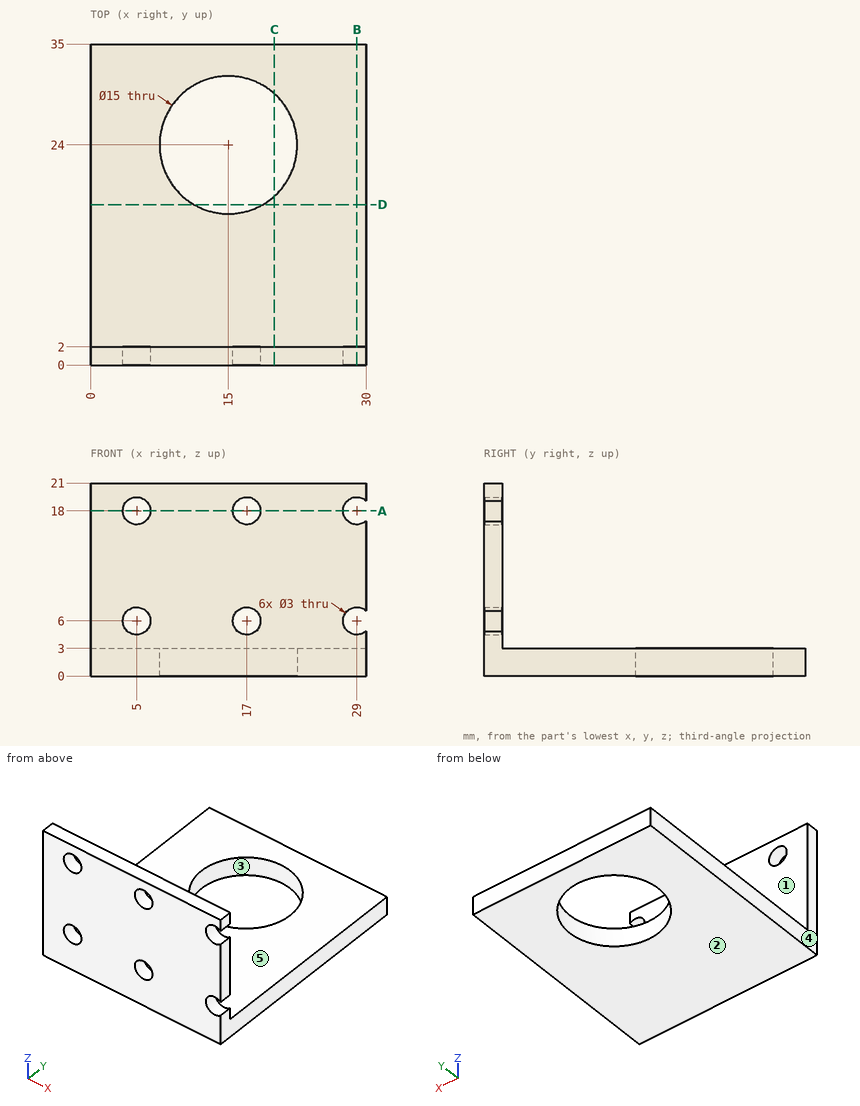
Print and shaded views of the part. All mm, measured from the part's lowest x, y and z. A direction names the side the tool comes from. Round coordinates to 2 decimals unless told otherwise and drop trailing zeros. Write each loop counter-clockwise with the first axis right and the second up, starting at its lowest first coordinate (ties: lowest second). Pieces come first, ordered by that corner, then holes. Notation, with made-up numbers: M 19.25,10 L 54.25,10 A16 cw 54.25,14 Z; hole C 11,82.5 d7. An arc over 180 degrees is marked long. Use a Markdown table: item, result. Add a question column.
1. Slice it at C-C on x = 20. Give the cut face in (y, z), then the cut area to 3 significant figures.
2. 3-axis set-ups, long thin cutter, end or side, ignore diameter. For the marked faces 4 and 5: which of +Z, -Z, +X, -X, +Y, -Y reach the whole face in a straight line?
3. Slice it at B-B on x = 29. Give the cut face in (y, z).
4. Slice it at A-A on z = 18. Give the cut face in (x, y), then the cut area to 3 significant figures.
5. Slice it at D-D on y = 17.5. Give the cut face in (x, z), then the cut area to 4 significant figures.
6. Flat gauge pins, fed straight in: P1, Ø5, axis at x = 17, z = 18, coming from the +Y side; P2, Ø5, axis at x = 24, y = 21.5, coming from the +Z side; P3, Ø2.5, axis at x = 5, z = 18, coming from the -Y side. Where does each tip first touch, or does it go through?
7. Pull direction Y, two halves, no side cores. Call the marked faces 1, 2 and 3: released by +Y, released by -Y, zero draft, split by the parting line, or undercut.
8. Drill centre lines: probe 1 along Z at (x, y) = (5, 1); probe 2 along X at (y, z) = (0.6, 18); probe 3 along Y at (x, z) = (15, 0.8). Where is each one in solid material? Low to high.
Reply:
| question | item | result |
|---|---|---|
| 1 | outline | M 0,0 L 18.41,0 L 18.41,3 L 2,3 L 2,21 L 0,21 Z; M 29.59,0 L 35,0 L 35,3 L 29.59,3 Z |
| 1 | area | 107 mm^2 |
| 2 | face 4 | +Z, -Z, -X, +Y, -Y |
| 2 | face 5 | +Z, +X, -X, +Y |
| 3 | outline | M 0,0 L 35,0 L 35,3 L 2,3 L 2,4.5 L 0,4.5 Z; M 0,7.5 L 2,7.5 L 2,16.5 L 0,16.5 Z; M 0,19.5 L 2,19.5 L 2,21 L 0,21 Z |
| 4 | outline | M 0,0 L 3.5,0 L 3.5,2 L 0,2 Z; M 6.5,0 L 15.5,0 L 15.5,2 L 6.5,2 Z; M 18.5,0 L 27.5,0 L 27.5,2 L 18.5,2 Z |
| 4 | area | 43.0 mm^2 |
| 5 | outline | M 0,0 L 11.26,0 L 11.26,3 L 0,3 Z; M 18.74,0 L 30,0 L 30,3 L 18.74,3 Z |
| 5 | area | 67.55 mm^2 |
| 6 | P1 | stops at y = 2 |
| 6 | P2 | stops at z = 3 |
| 6 | P3 | passes through |
| 7 | face 1 | released by +Y |
| 7 | face 2 | zero draft |
| 7 | face 3 | undercut |
| 8 | probe 1 | z = 0 to 4.5, 7.5 to 16.5, 19.5 to 21 |
| 8 | probe 2 | x = 0 to 3.5, 6.5 to 15.5, 18.5 to 27.5 |
| 8 | probe 3 | y = 0 to 16.5, 31.5 to 35 |
